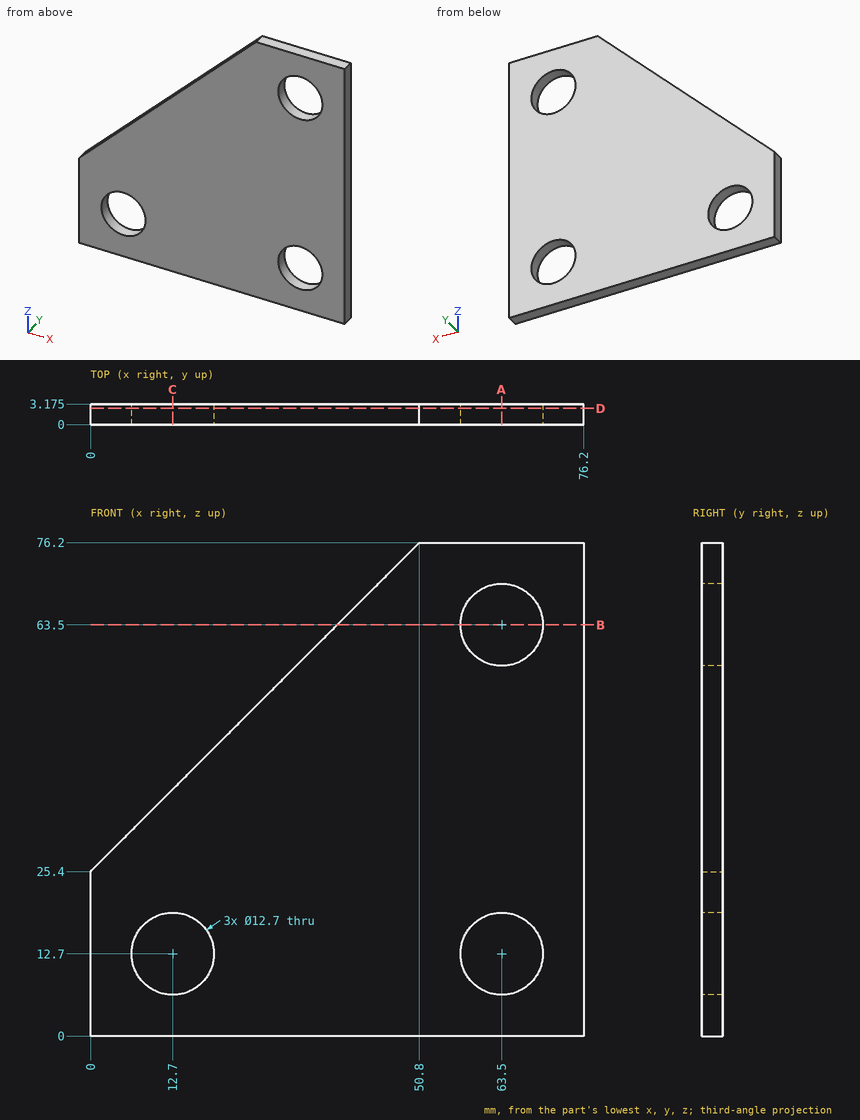
Answer from the drawing. Dimensions are ordinates in mm from the lowest x, y and z of the part. Give positions to 0.01 mm unless a question says otherwise; leave off trailing zeros. Order: outer loops, then holes, each group sorted by start corner. A loop starts at its lowest first (then second) coordinate and runs counter-clockwise, first axis right, second up.
Item 1: The part is cut by section D-D, the plane y = 2.5. Give the vertices of the cut face in (x, z).
From the geometry:
outline: (0, 0) - (76.2, 0) - (76.2, 76.2) - (50.8, 76.2) - (0, 25.4) - close; hole circle Ø12.7 at (12.7, 12.7); hole circle Ø12.7 at (63.5, 12.7); hole circle Ø12.7 at (63.5, 63.5)
Item 2: The part is cut by section A-A, the plane x = 63.5. Give the vertices of the cut face in (y, z) (3 decimals), and give its area (3 significant figures).
From the geometry:
outline: (0, 0) - (3.175, 0) - (3.175, 6.35) - (0, 6.35) - close; (0, 19.05) - (3.175, 19.05) - (3.175, 57.15) - (0, 57.15) - close; (0, 69.85) - (3.175, 69.85) - (3.175, 76.2) - (0, 76.2) - close
area: 161 mm2
Item 3: Find the intervals of material crossed by probe 1 along Z at (x, y) = (63.5, 2.2); probe 2 along X at (y, z) = (1, 15); probe 3 along Z at (x, y) = (8, 2.15), in increasing order.
From the geometry:
probe 1: z = 0 to 6.35, 19.05 to 57.15, 69.85 to 76.2
probe 2: x = 0 to 6.78, 18.62 to 57.58, 69.42 to 76.2
probe 3: z = 0 to 8.43, 16.97 to 33.4
Item 4: Given pin 1 Ø1.5 at (y, z) = (0.5, 62.5) entering from -X; pin 2 Ø12 at (x, z) = (13.5, 46) entering from +Y (3 decimals); pin 3 Ø1.5 at (y, z) = (2, 54.5) entering from -X; pin 4 Ø1.5 at (x, y) = (40.5, 0.5) entering from +Z, each flat-ended and moving along its own axis, determine where each tip first touches the part or whether it passes through.
From the geometry:
pin 1: stops at x = 36.35
pin 2: stops at y = 3.175
pin 3: stops at x = 28.35
pin 4: stops at z = 66.65
Item 5: The part is cut by section B-B, the plane z = 63.5. Give the vertices of the cut face in (x, y) (3 decimals).
From the geometry:
outline: (38.1, 0) - (57.15, 0) - (57.15, 3.175) - (38.1, 3.175) - close; (69.85, 0) - (76.2, 0) - (76.2, 3.175) - (69.85, 3.175) - close
Item 6: The part is cut by section C-C, the plane x = 12.7. Give the vertices of the cut face in (y, z) (3 decimals), and give its area (3 significant figures).
From the geometry:
outline: (0, 0) - (3.175, 0) - (3.175, 6.35) - (0, 6.35) - close; (0, 19.05) - (3.175, 19.05) - (3.175, 38.1) - (0, 38.1) - close
area: 80.6 mm2
